Input: dimensioned drawing with shaded views. Units: mm. Origin: part minimum x, y, z. A direction names the side the tool comes from. Round coordinates to 2 decimals unless told otherwise and drop trailing zeros. Loops run counter-clockwise (first coordinate to the right, second up) from the corner with the lowest first, then second, coordinate; pieces in that order, holes last. Notation, with made-up numbers: M 18,15 L 66,15 A22 cw 66,31 Z; hole C 69,-37.75 d8. An arc over 180 degrees is marked long. Put each result on its own line as item: value. Start each with the question number.
1) Pin query (flat end, axial travel): pin 1 (10 mm diameter, centred on y = 37.5, z = 31.5, fed in from +X); pin 2 (16.5 mm diameter, centred on x = 61.5, z = 37.5, fed in from -Y); pin 3 (21.5 mm diameter, centred on x = 29, y = 28, fed in from +Z); pin 4 (6 mm diameter, centred on x = 102.5, z = 18.5, fed in from -Y) (1 decimal). Return the tip coordinate at first contact, or that it passes through.
2) Section A-A on y = 3. Output: boundary loops of the cut face in (x, z) (1 decimal).
3) Section D-D on y = 34.5. Output: boundary loops of the cut face in (x, z) (1 decimal), plus the area to 3 significant figures.
4) Section B-B on z = 16. Output: boundary loops of the cut face in (x, y), plus the area to 3 significant figures.
5) Reachability of the marked faces 4, 5, 6 and 7 from +Z, -Z, +X, -X, +Y, -Y: full face, straight path, thin tool, end or side. Return the list, or none.
6) Section C-C on x = 42. Output: boundary loops of the cut face in (y, z).
7) Draft query along X for the marked faces 1, 2 and 3. Return one class per face: +X half, -X half, draft (parallel to the pull), parting line (faces both ways), or undercut.
8) Line query: probe 1 along Z at (x, y) = (11.5, 29) (1 decimal); probe 2 along X at (y, z) = (25, 33); probe 3 along Z at (x, y) = (87.5, 6). Output: solid intervals per line, ascending.
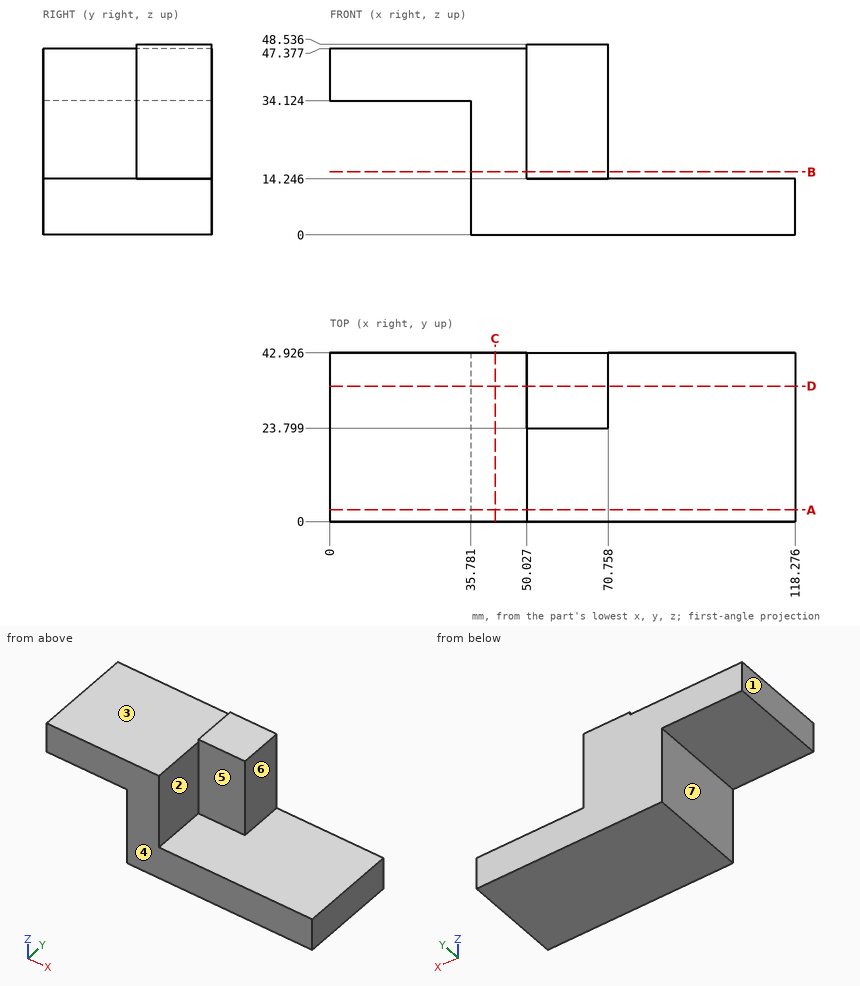
Geometry results:
1. pin 1: stops at x = 70.76
1. pin 2: stops at y = 23.8
1. pin 3: stops at z = 47.38
1. pin 4: passes through
2. outline: M 0,34.1 L 35.8,34.1 L 35.8,0 L 118.3,0 L 118.3,14.2 L 50,14.2 L 50,47.4 L 0,47.4 Z
3. outline: M 0,34.1 L 35.8,34.1 L 35.8,0 L 118.3,0 L 118.3,14.2 L 70.8,14.2 L 70.8,48.5 L 50,48.5 L 50,47.4 L 0,47.4 Z
3. area: 2,830 mm²
4. outline: M 35.78,0 L 50.03,0 L 50.03,23.8 L 70.76,23.8 L 70.76,42.93 L 35.78,42.93 Z
4. area: 1,010 mm²
5. face 4: +Z, -Z, +X, -X, -Y
5. face 5: +Z, +X, -Y
5. face 6: +Z, +X, +Y, -Y
5. face 7: -Z, -X, +Y, -Y
6. outline: M 0,0 L 42.93,0 L 42.93,47.38 L 0,47.38 Z
7. face 1: -X half
7. face 2: +X half
7. face 3: draft
8. probe 1: z = 34.1 to 47.4
8. probe 2: x = 35.78 to 70.76
8. probe 3: z = 0 to 14.25
